Part model, mm, in its own coordinate system. A direction names the side the tool comes from. Give positions to 0.01 mm unless a question says otherwise; leave off trailing zeros. Write each loop counter-clockwise with the first axis right and the second up, starting at its lowest first coordinate (ties: lowest second). Pieces come first, ordered by that corner, then holes. Notation, with made-up numbers: M -9,51 L 38,51 A23 ccw 38,76 Z; hole C 44,3.5 d11. An arc over 180 degrees is marked long. Use a Markdown table: item, result.
```python
from build123d import *

# Parameters (mm, degrees)
SKETCH1_R           = 1.5
BOSS_EXTRUDE1_DEPTH = 3
FILLET1_R           = 2
SKETCH3_W           = 20
SKETCH3_H           = 42
BOSS_EXTRUDE2_DEPTH = 8
FILLET2_R           = 2
SKETCH4_R           = 9.99
CUT_EXTRUDE1_DEPTH  = 12
SKETCH5_R           = 1.5
CUT_EXTRUDE2_DEPTH  = 49


with BuildPart() as part:
    # Sketch1 → Boss-Extrude1 (new body)
    with BuildSketch(Plane.XY):
        Polygon((12, 22.5), (7.96, 22.5), (7.96, 27), (1.96, 27), (1.96, 22.5), (-12, 22.5), (-12, -22.5), (-7.96, -22.5), (-7.96, -27), (-1.96, -27), (-1.96, -22.5), (12, -22.5), align=None)
        with Locations((4.96, 24)):
            Circle(SKETCH1_R, mode=Mode.SUBTRACT)
        with Locations((-4.96, -24)):
            Circle(SKETCH1_R, mode=Mode.SUBTRACT)
    extrude(amount=BOSS_EXTRUDE1_DEPTH)

    # Fillet1
    fillet1_edges = [part.edges().sort_by_distance(p)[0] for p in [
        (-12, 22.5, 1.5),
        (12, 22.5, 1.5),
        (12, -22.5, 1.5),
        (-12, -22.5, 1.5),
    ]]
    fillet(fillet1_edges, radius=FILLET1_R)

    # Sketch3 → Boss-Extrude2 (add)
    with BuildSketch(Plane.XY.offset(3)):
        Rectangle(SKETCH3_W, SKETCH3_H)
    extrude(amount=BOSS_EXTRUDE2_DEPTH)

    # Fillet2
    fillet2_edges = [part.edges().sort_by_distance(p)[0] for p in [
        (-10, 21, 7),
        (-10, -21, 7),
        (10, -21, 7),
        (10, 21, 7),
    ]]
    fillet(fillet2_edges, radius=FILLET2_R)

    # Sketch4 → Cut-Extrude1 (cut, through all)
    with BuildSketch(Plane.XY.offset(11)):
        with Locations((0, 9)):
            Circle(SKETCH4_R)
    extrude(amount=-CUT_EXTRUDE1_DEPTH, mode=Mode.SUBTRACT)

    # Sketch5 → Cut-Extrude2 (cut, through all)
    with BuildSketch(Plane(origin=(0, 21, 0), x_dir=(1, 0, 0), z_dir=(0, 1, 0))):
        with Locations((0.05, -4.5)):
            Circle(SKETCH5_R)
    extrude(amount=-CUT_EXTRUDE2_DEPTH, mode=Mode.SUBTRACT)


solid = part.part
```
1. Cut at B-B, the plane x = -4.96. Give the cut face in (y, z), then the cut area to 3 significant figures.
Findings below:
| item | result |
|---|---|
| outline | M -27,0 L -25.5,0 L -25.5,3 L -27,3 Z; M -22.5,0 L 0.33,0 L 0.33,11 L -21,11 L -21,3 L -22.5,3 Z; M 17.67,0 L 22.5,0 L 22.5,3 L 21,3 L 21,11 L 17.67,11 Z |
| area | 285 mm2 |
2. Drop flat-ended pins along their axis: P1, Ø2.5, axis at y = -24, z = 1, coming from the +X side; P2, Ø4, axis at y = -1.5, z = 8, coming from the +X side; P3, Ø1.5, axis at x = -6, z = 2, coming from the +Y side. Give the stop position or say it passes through.
Findings below:
| item | result |
|---|---|
| P1 | x = -1.96 |
| P2 | x = 10 |
| P3 | y = 22.5 |
3. Drill centre lines: L1, parallel to Y at x = -0.25, z = 10.5; L2, parallel to Z at x = 0.05, y = -5.5; L3, parallel to Z at x = 10.5, y = 13. Where is each one in solid material? Low to high.
Findings below:
| item | result |
|---|---|
| L1 | -21 to -0.99, 18.99 to 21 |
| L2 | 0 to 3, 6 to 11 |
| L3 | 0 to 3 |
4. Two-plate mould, pull along Y, no slides. Class faces 4 (the flat face through (-7.96, -25, 1)), 5 (the flat face through (0, -21, 7)), 6 (the cylindrical face through (4.765, 25.487, 1.479)): released by +Y, released by -Y, zero draft, split by the parting line, or undercut.
Findings below:
| item | result |
|---|---|
| face 4 | zero draft |
| face 5 | released by -Y |
| face 6 | undercut |
5. Tool access for faces 1 (the flat face through (-10, 0, 7)), 2 (the flat face through (0, 21, 7)), 3 (the flat face through (1.96, 25, 1)): list every direction of +Z, -Z, +X, -X, +Y, -Y with a clear straight run to the whole face (end or side of a thin tool).
Findings below:
| item | result |
|---|---|
| face 1 | +Z, -X, +Y, -Y |
| face 2 | +Z, +X, -X, +Y |
| face 3 | +Z, -Z, -X, +Y |
6. Cut at D-D, the plane z = 7.5. Give the cut face in (x, y).
Findings below:
| item | result |
|---|---|
| outline | M -10,-19 A2 ccw -8,-21 L 8,-21 A2 ccw 10,-19 L 10,19 A2 ccw 8,21 L -8,21 A2 ccw -10,19 Z; hole C 0,9 d19.98 |
7. Cut at C-C, the plane z = 1. Give the cut face in (x, y), then the cut area to 3 significant figures.
Findings below:
| item | result |
|---|---|
| outline | M -12,-20.5 A2 ccw -10,-22.5 L -7.96,-22.5 L -7.96,-27 L -1.96,-27 L -1.96,-22.5 L 10,-22.5 A2 ccw 12,-20.5 L 12,20.5 A2 ccw 10,22.5 L 7.96,22.5 L 7.96,27 L 1.96,27 L 1.96,22.5 L -10,22.5 A2 ccw -12,20.5 Z; hole C 0,9 d19.98; hole C -4.96,-24 d3; hole C 4.96,24 d3 |
| area | 803 mm2 |
8. Cut at A-A, the plane y = -24. Give the cut face in (x, z), then the cut area to 3 significant figures.
Findings below:
| item | result |
|---|---|
| outline | M -7.96,0 L -6.46,0 L -6.46,3 L -7.96,3 Z; M -3.46,0 L -1.96,0 L -1.96,3 L -3.46,3 Z |
| area | 9.00 mm2 |
